Answer from the drawing. Dimensions are ordinates in mm from the lowest x, y and z of the part. Coordinates: 2 decimals unless noted, no trailing zeros. Write each loop counter-clockwise with the first axis right and the second up, starting at its lowest first coordinate (ties: lowest second). Pieces come first, ordered by that corner, then holes. Notation, with made-up numbers: (50.25, -38) - (102.25, -38) arc R34 cw to (102.25, -8) - close; hole circle Ø7 at (41, 72). An arc over 180 degrees is marked (long way). Use CSV: the item, a comma, the result in double quotes. Start each with the question number.
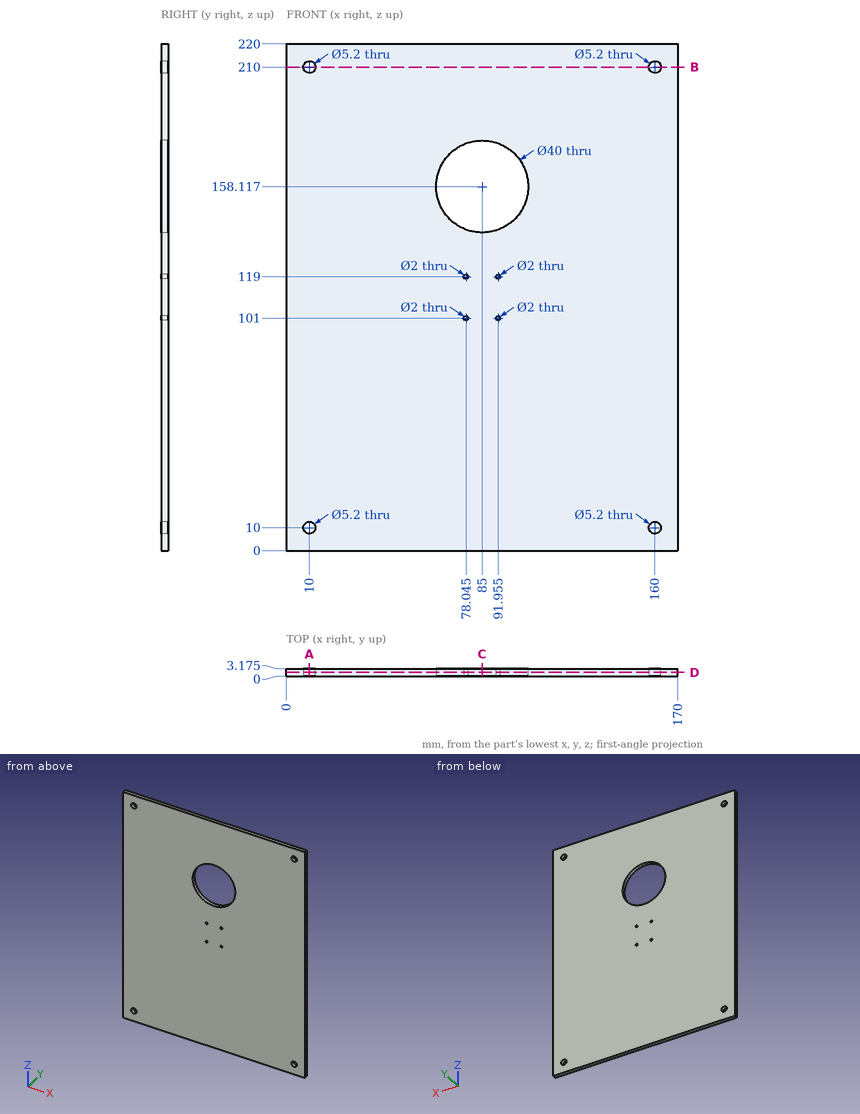
Item 1: A cutting plane is placed at A-A (x = 10). Determine the outline of the cut face in (y, z) (1 decimal).
Item 2: A cutting plane is placed at C-C (x = 85). Determine the outline of the cut face in (y, z) (1 decimal).
Item 3: A cutting plane is placed at D-D (y = 1.6). Count the separate pieces of the cut face and the enclosed holes in it, then the cut area to 3 significant figures.
Item 4: Straight lines are drawn through the part: probe 1 along X at (y, z) = (0.8, 119) (1 decimal); probe 2 along Z at (x, y) = (10, 0.85); probe 3 along Z at (x, y) = (161, 2.8). For each, find the intervals that lie inside material, in ascending order. Write a range as [from, to].
Item 5: A cutting plane is placed at B-B (z = 210). Determine the outline of the cut face in (x, y) (1 decimal).
Item 6: This flat-tipped pin is pushed along its axis until it touches: pin 1 (3 mm diameter, centred on x = 10, z = 210, fed in from -Y). Where does it stop, or does it pass through?
Calculated:
1,outline,"(0, 0) - (3.2, 0) - (3.2, 7.4) - (0, 7.4) - close; (0, 12.6) - (3.2, 12.6) - (3.2, 207.4) - (0, 207.4) - close; (0, 212.6) - (3.2, 212.6) - (3.2, 220) - (0, 220) - close"
2,outline,"(0, 0) - (3.2, 0) - (3.2, 138.1) - (0, 138.1) - close; (0, 178.1) - (3.2, 178.1) - (3.2, 220) - (0, 220) - close"
3,separate pieces,"1"
3,enclosed holes,"9"
3,area,"36,000 mm²"
4,probe 1,"x = [0, 77], [79, 91], [93, 170]"
4,probe 2,"z = [0, 7.4], [12.6, 207.4], [212.6, 220]"
4,probe 3,"z = [0, 7.6], [12.4, 207.6], [212.4, 220]"
5,outline,"(0, 0) - (7.4, 0) - (7.4, 3.2) - (0, 3.2) - close; (12.6, 0) - (157.4, 0) - (157.4, 3.2) - (12.6, 3.2) - close; (162.6, 0) - (170, 0) - (170, 3.2) - (162.6, 3.2) - close"
6,pin 1,"passes through"
